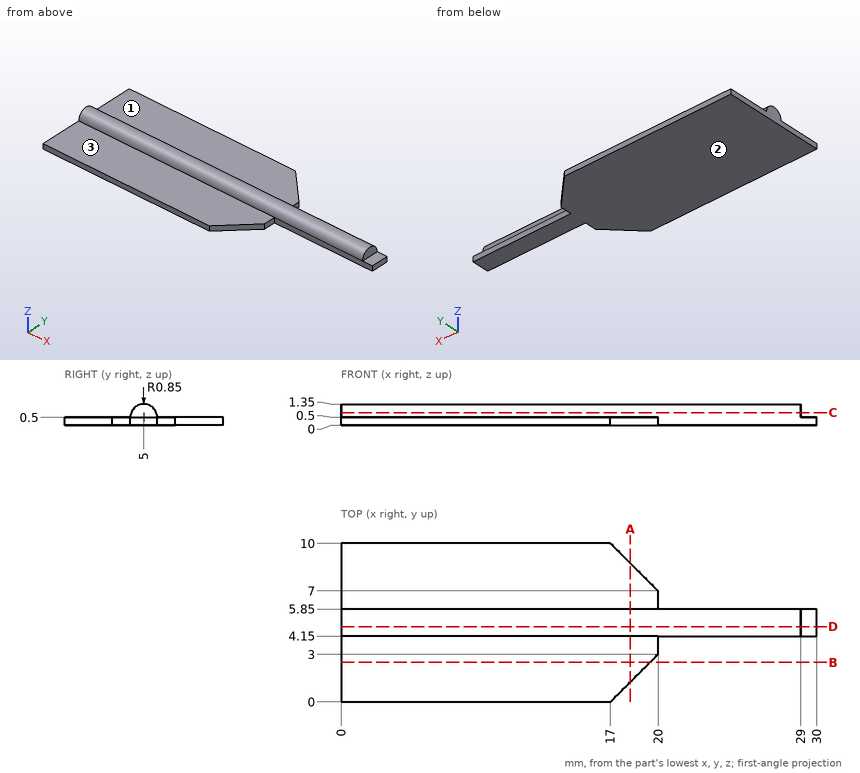
Geometry check sheet. Reference: drawing and pictorial views, mm from the part's lowest x, y, z. A direction names the side the tool comes from. Give positions to 0.01 mm unless a question says otherwise; leave off trailing zeros. Order: outer loops, then holes, each group sorted by start corner. A loop starts at its lowest first (then second) coordinate and runs counter-clockwise, first axis right, second up. Notation, with made-up numbers: M 34.25,75 L 79.25,75 A15 ccw 79.25,89 Z; hole C 28.25,-3.75 d8. An arc over 180 degrees is marked long. Answer in a Markdown table with one row per item.
1) Thickness scan on L1, parallel to Z at x = 14, y = 3.5; L2, parallel to Y at x = 26, z = 0.55; L3, parallel to X at y = 5, z = 0.9. Record the ranges inside material, lowest first. Write a range as [from, to].
Filled sheet:
| item | result |
|---|---|
| L1 | z = [0, 0.5] |
| L2 | y = [4.15, 5.85] |
| L3 | x = [0, 29] |
2) Cross-section at D-D, the plane y = 4.75. Enter the section's corners in (x, z), plus the area to 3 significant figures.
Filled sheet:
| item | result |
|---|---|
| outline | M 0,0 L 30,0 L 30,0.5 L 29,0.5 L 29,1.31 L 0,1.31 Z |
| area | 38.6 mm2 |
3) Cross-section at A-A, the plane x = 18.25. Enter the section's corners in (y, z).
Filled sheet:
| item | result |
|---|---|
| outline | M 1.25,0 L 8.75,0 L 8.75,0.5 L 5.85,0.5 A0.85 ccw 4.15,0.5 L 1.25,0.5 Z |
4) Gauge pin test, flat ends, axial feed: P1, Ø2, axis at x = 3, y = 9, coming from the +Z side; P2, Ø1.1, axis at x = 29.5, y = 5, coming from the +Z side. Record the tip position at first contact, or that the pin passes through.
Filled sheet:
| item | result |
|---|---|
| P1 | stops at z = 0.5 |
| P2 | stops at z = 1.35 |
5) Access from +Z, -Z, +X, -X, +Y, -Y to the whole of each face (thin tool, end or side, straight path). Record for the marked faces 1, 2 and 3.
Filled sheet:
| item | result |
|---|---|
| face 1 | +Z, +X, -X, +Y |
| face 2 | -Z, +X, -X, +Y, -Y |
| face 3 | +Z, +X, -X, -Y |
6) Cross-section at C-C, the plane z = 0.8. Enter the section's corners in (x, y).
Filled sheet:
| item | result |
|---|---|
| outline | M 0,4.2 L 29,4.2 L 29,5.8 L 0,5.8 Z |
7) Cross-section at B-B, the plane y = 2.5. Enter the section's corners in (x, z), plus the area to 3 significant figures.
Filled sheet:
| item | result |
|---|---|
| outline | M 0,0 L 19.5,0 L 19.5,0.5 L 0,0.5 Z |
| area | 9.75 mm2 |
